Autodesk Inventor part; units mm, degrees
ref_plane "YZ Plane" through (0, 0, 0) normal (1, 0, 0) x (0, 1, 0)
ref_plane "XZ Plane" through (0, 0, 0) normal (0, 1, 0) x (-1, 0, 0)
ref_plane "XY Plane" through (0, 0, 0) normal (0, 0, 1) x (1, 0, 0)
sketch "Sketch1" plane through (0, 0, 0) normal (0, 0, 1) x (1, 0, 0)
  line L0 (6.0325, -17.78) -> (-6.0325, -17.78)
  line L1 (-6.0325, -17.78) -> (-6.0325, 17.78)
  line L2 (-6.0325, 17.78) -> (6.0325, 17.78)
  line L3 (6.0325, 17.78) -> (6.0325, -17.78)
  line L4 (6.0325, -17.78) -> (-6.0325, 17.78) construction
  line L5 (-6.0325, -17.78) -> (6.0325, 17.78) construction
  point P0 (0, 0)
  dimension "d0" = 12.065
  dimension "d1" = 35.56
extrude "Extrusion1" add sketch "Sketch1" along normal blind 25.4
sketch "Sketch3" plane through (0, 0, 25.4) normal (0, 0, 1) x (1, 0, 0)
  line L0 (6.0325, -17.78) -> (6.0325, 17.78)
  line L1 (0, 26.67) -> (0, -26.67)
  line L2 (-8.4455, 0) -> (8.4455, 0)
  point P0 (0, 12.7)
  point P1 (0, -12.7)
  dimension "d45" = 12.7
  dimension "d46" = 12.7
  dimension "d47" = 0
hole "Hole5" at (0, 12.7, 25.4) at (0, -12.7, 25.4) direction (0, 0, -1) diameter 3.2512 depth 11.811 tip angle 118
sketch "Sketch7" plane through (0, 0, 0) normal (0, 0, -1) x (-1, 0, 0)
  line L0 (-6.0325, -17.78) -> (6.0325, -17.78)
  line L1 (6.0325, 17.78) -> (-6.0325, 17.78)
  line L2 (-6.0325, 17.78) -> (-6.0325, -17.78)
  line L3 (-15.0439, 0) -> (-8.5725, -17.78)
  line L4 (-6.0325, -17.78) -> (-8.5725, -17.78)
  line L5 (-15.0439, 0) -> (-8.5725, 17.78)
  line L6 (-8.5725, 17.78) -> (-6.0325, 17.78)
  line L7 (0, -26.67) -> (0, 26.67)
  line L8 (-19.0666, 0) -> (10.2157, 0)
  point P0 (0, 0)
  dimension "d70" = 70
  dimension "d71" = 70
  dimension "d72" = 2.54
extrude "Extrusion6" add sketch "Sketch7" against normal blind 5.08 contours L4 L3 L8 L2 | L8 L5 L6 L2
fillet "Fillet1" radius 3.175 1 edges at (15.0439, 0, 2.54)
fillet "Fillet2" radius 1.27 2 edges at (8.5725, -17.78, 2.54) (8.5725, 17.78, 2.54)
chamfer "Chamfer1" distance 8.255 angle 45 1 edges at (-6.0325, 0, 0)
sketch "Sketch8" plane through (0, 0, 0) normal (0, 0, -1) x (-1, 0, 0)
  line L0 (-2.2225, 17.78) -> (-2.2225, -17.78)
  line L1 (-2.2225, 17.78) -> (-7.6832, 17.78)
  arc A0 (-7.6832, 17.78) -> (-8.8766, 16.9444) centre (-7.6832, 16.51) ccw
  line L2 (-8.8766, 16.9444) -> (-14.6487, 1.0859)
  arc A1 (-14.6487, 1.0859) -> (-14.6487, -1.0859) centre (-11.6651, 0) ccw
  line L3 (-14.6487, -1.0859) -> (-8.8766, -16.9444)
  arc A2 (-8.8766, -16.9444) -> (-7.6832, -17.78) centre (-7.6832, -16.51) ccw
  line L4 (-7.6832, -17.78) -> (-2.2225, -17.78)
  line L5 (-14.6487, 1.0859) -> (-8.8766, 16.9444)
  line L6 (-13.8951, 3.1562) -> (-6.2749, -17.78)
  line L7 (-14.6487, -1.0859) -> (-8.8766, -16.9444)
  point P0 (0, 0)
  dimension "d80" = 2.159
extrude "Extrusion7" cut sketch "Sketch8" against normal up to next contours L4 A2 L3 A1 L2 L6
properties part number "J005413" material "ALUMINUM, 6061-T651"
Part model, mm, in its own coordinate system. A direction names the side the tool comes from. Round coordinates to 2 decimals unless told otherwise and drop trailing zeros. Loops run counter-clockwise (first coordinate to the right, second up) from the corner with the lowest first, then second, coordinate; pieces in that order, holes last.
1. 3-axis set-ups, long thin cutter, end or side, ignore diameter. For faces 1 (the face through (0, 0, 25.4)), 2 (the face through (-0.071, -11.076, 19.412)), 3 (the face through (9, 4, 5.08)): which of +Z, -Z, +X, -X, +Y, -Y reach the whole face in a straight line?
Solutions:
face 1: +Z, +X, -X, +Y, -Y
face 2: +Z
face 3: +Z, +X, +Y, -Y
2. Slice it at C-C (z = 9). Give the cut face in (x, y).
Solutions:
outline: (-6.03, -17.78) - (6.03, -17.78) - (6.03, 17.78) - (-6.03, 17.78) - close
3. Slice it at B-B (y = 1). Give the cut face in (x, z) (1 decimal).
Solutions:
outline: (-6, 8.3) - (2.2, 0) - (13.1, 0) - (13.1, 5.1) - (6, 5.1) - (6, 25.4) - (-6, 25.4) - close
4. Drill centre lines: line 1 along Y through (x, z) = (0, 19.75); line 2 along X through (y, z) = (12.7, 16.5); line 3 along X through (y, z) = (-11, 12.25). Where is each one in solid material? Low to high.
Solutions:
line 1: y = -17.78 to -14.33, -11.07 to 11.07, 14.33 to 17.78
line 2: x = -6.03 to -1.63, 1.63 to 6.03
line 3: x = -6.03 to 6.03
5. Slice it at D-D (y = -6). Give the cut face in (x, z) (1 decimal), and give its area (3 significant figures).
Solutions:
outline: (-6, 8.3) - (2.2, 0) - (10.6, 0) - (10.6, 5.1) - (6, 5.1) - (6, 25.4) - (-6, 25.4) - close
area: 295 mm2
6. Slice it at A-A (z = 22.25). Give the cut face in (x, y), and give its area (3 significant figures).
Solutions:
outline: (-6.03, -17.78) - (6.03, -17.78) - (6.03, 17.78) - (-6.03, 17.78) - close; hole circle Ø3.25 at (0, -12.7); hole circle Ø3.25 at (0, 12.7)
area: 412 mm2
7. Flat gauge pins, fed straight in: pin 1 (6.5 mm diameter, centred on x = 10.5, y = 4.5, fed in from +Z); pin 2 (3.5 mm diameter, centred on x = 0, y = -12.7, fed in from -Z); pin 3 (1 mm diameter, centred on y = 10, z = 19, fed in from +X). Where does each tip first touch, or does it go through?
Solutions:
pin 1: stops at z = 5.08
pin 2: stops at z = 0.47
pin 3: stops at x = 6.03
8. Two-plate mould, pull along Y, no slides. Class faces 4 (the face through (11.421, 9.954, 2.504)), 5 (the face through (0, -17.78, 13)), 6 (the face through (0.623, 11.198, 19.412)), 7 (the face through (0.01, -12.42, 12.78)): pulls with the +Y half, pulls with the -Y half, needs draft (parallel to the pull), parting line crosses it, or undercut.
Solutions:
face 4: pulls with the +Y half
face 5: pulls with the -Y half
face 6: undercut
face 7: undercut
